```python
from build123d import *

# Parameters (mm, degrees)
F0_W        = 78
F0_H        = 38
F1_DEPTH    = 4
F2_W        = 78
F2_H        = 3
F3_DEPTH    = 81
F4_T1_DEPTH = 203
F5_R        = 31
F5_R_2      = 29.5
F6_DEPTH    = 27
F7_R        = 28.5
F8_DEPTH    = 3
F9_R        = 31
F10_DEPTH   = 2
F11_R       = 16
F12_DEPTH   = 2
F14_DEPTH   = 4


# Not quite as in the source:
# - a fillet or chamfer that OpenCascade refuses, or shapes differently, is made with other operations: its cross-section is extruded or revolved along the edge and cut away or added


with BuildPart() as f1:
    # F0 (on Top) → F1 (new body)
    with BuildSketch(Plane.XY):
        Rectangle(F0_W, F0_H)
    extrude(amount=F1_DEPTH)

    # F2 (on face) → F3 (join)
    with BuildSketch(Plane.XY.offset(4)):
        with Locations((0, 17.5)):
            Rectangle(F2_W, F2_H)
    extrude(amount=F3_DEPTH)

    # F4: fillet of radius 40 on 2 edges, made by hand

    # F4_s2 → F4_t1 (cut)
    with BuildSketch(Plane.XZ.offset(-119)):
        with BuildLine():
            ThreePointArc((39, 45), (27.2842712475, 73.2842712475), (-1, 85))
            Line((-1, 85), (39, 85))
            Line((39, 85), (39, 45))
        make_face()
        with BuildLine():
            ThreePointArc((-39, 45), (-27.2842712475, 73.2842712475), (1, 85))
            Line((1, 85), (-39, 85))
            Line((-39, 85), (-39, 45))
        make_face()
    extrude(amount=F4_T1_DEPTH, mode=Mode.SUBTRACT)

    # F5 (on face) → F6 (join)
    with BuildSketch(Plane(origin=(0, 19, 0), x_dir=(-1, 0, 0), z_dir=(0, 1, 0))):
        with Locations((0, 45.9753048304)):
            Circle(F5_R)
        with Locations((0, 45.9753048304)):
            Circle(F5_R_2, mode=Mode.SUBTRACT)
    extrude(amount=F6_DEPTH)

    # F7 (on face) → F8 (cut, through all)
    with BuildSketch(Plane(origin=(0, 19, 0), x_dir=(-1, 0, 0), z_dir=(0, 1, 0))):
        with Locations((0, 45.9753048304)):
            Circle(F7_R)
    extrude(amount=-F8_DEPTH, mode=Mode.SUBTRACT)

    # F9 (on face) → F10 (join)
    with BuildSketch(Plane(origin=(0, 46, 0), x_dir=(-1, 0, 0), z_dir=(0, 1, 0))):
        with Locations((0, 45.9753048304)):
            Circle(F9_R)
    extrude(amount=F10_DEPTH)

    # F11 (on face) → F12 (cut, through all)
    with BuildSketch(Plane(origin=(0, 48, 0), x_dir=(-1, 0, 0), z_dir=(0, 1, 0))):
        with Locations((0, 45.9753048304)):
            Circle(F11_R)
    extrude(amount=-F12_DEPTH, mode=Mode.SUBTRACT)

    # F13 (on face) → F14 (cut, through all)
    with BuildSketch(Plane.XY.offset(4)):
        with BuildLine():
            Line((29.2, -19), (33.7, -19))
            Line((33.7, -19), (33.7, -9))
            ThreePointArc((33.7, -9), (31.45, -11.25), (29.2, -9))
            Line((29.2, -9), (29.2, -19))
        make_face()
        with BuildLine():
            ThreePointArc((29.2, -9), (31.45, -11.25), (33.7, -9))
            Line((33.7, -9), (29.2, -9))
        make_face()
        with BuildLine():
            Line((29.2, -9), (33.7, -9))
            ThreePointArc((33.7, -9), (31.45, -6.75), (29.2, -9))
        make_face()
        with BuildLine():
            ThreePointArc((-29.2, -9), (-31.45, -6.75), (-33.7, -9))
            Line((-33.7, -9), (-29.2, -9))
        make_face()
        with BuildLine():
            ThreePointArc((-29.2, -9), (-31.45, -11.25), (-33.7, -9))
            Line((-33.7, -9), (-33.7, -19))
            Line((-33.7, -19), (-29.2, -19))
            Line((-29.2, -19), (-29.2, -9))
        make_face()
        with BuildLine():
            Line((-29.2, -9), (-33.7, -9))
            ThreePointArc((-33.7, -9), (-31.45, -11.25), (-29.2, -9))
        make_face()
    extrude(amount=-F14_DEPTH, mode=Mode.SUBTRACT)


solid = f1.part
```
The listing builds one solid part. Answer for the finished solid, in the listing's coordinates (mm). A direction names the side the tool comes from. Give positions to 0.01 mm unless a question says otherwise; leave off trailing zeros. Write each loop counter-clockwise with the first axis right and the second up, starting at its lowest first coordinate (ties: lowest second). Pieces come first, ordered by that corner, then holes. Notation, with made-up numbers: M -30.5,82.25 L -18.5,82.25 A35 cw -18.5,115.25 Z; hole C 16.5,31 d4. An arc over 180 degrees is marked long. Write each question's results on one line, items separated by ' | '.
Q1. A tool of negligible diameter and unlimited length cuts with its end or side. For faces 5 (the flat face through (-1, -1, 4)), 6 (the cylindrical face through (6.72, 33.297, 15.712)), 7 (the flat face through (33.7, -14, 2)), from which of +Z, -Z, +X, -X, +Y, -Y can it reach the whole face along a straight path? Write none if from no direction.
Output values:
face 5: +Z, +X, -X, -Y | face 6: +Y | face 7: +Z, -Z, -Y
Q2. Section B-B, the plane x = 3.5 is taken. Write down the section's boundary in (y, z).
Output values:
outline: M -19,0 L 19,0 L 19,15.17 L 48,15.17 L 48,30.36 L 46,30.36 L 46,16.68 L 19,16.68 L 19,17.69 L 16,17.69 L 16,4 L -19,4 Z; M 16,74.26 L 19,74.26 L 19,75.27 L 46,75.27 L 46,61.59 L 48,61.59 L 48,76.78 L 19,76.78 L 19,84.75 L 16,84.75 Z
Q3. For a pull along Y with two mould halves and no side action, classify faces 1 (the cylindrical face through (6.395, 32.311, 17.177)), 2 (the flat face through (-29.2, -14, 2)), 3 (the flat face through (-1, 16, 17)), 4 (the flat face through (-13, 48, 33)) as released by +Y, released by -Y, zero draft, split by the parting line, or undercut.
Output values:
face 1: undercut | face 2: zero draft | face 3: released by -Y | face 4: released by +Y
Q4. Consider L1, parallel to Z at x = 0, y = 46.7; L2, parallel to Z at x = 0, y = 17.05; L3, parallel to Z at x = 4, y = -15. Determine where each line is inside the solid, lowest interval first. Write a range as from..to.
Output values:
L1: 14.98..29.98, 61.98..76.98 | L2: 0..17.48, 74.48..84.99 | L3: 0..4
Q5. Section C-C, the plane y = -5.5 is taken. Write down the section's boundary in (x, z), then the cut area to 3 significant figures.
Output values:
outline: M -39,0 L 39,0 L 39,4 L -39,4 Z | area: 312 mm2
Q6. Flat-ended cylindrical pins translate along their axes: P1, Ø1.5, axis at x = 0.5, y = -11, coming from the +Z side; P2, Ø5, axis at x = 29, z = 21, coming from the +Y side; P3, Ø6, axis at x = -21, y = 27, coming from the +Z side. Find the tip coordinate at first contact, or state that the pin passes through.
Output values:
P1: z = 4 | P2: y = 19 | P3: z = 71.21
Q7. Section A-A, the plane z = 40.5 is taken. Write down the section's boundary in (x, y), then the cut area to 3 significant figures.
Output values:
outline: M -39,16 L -27.97,16 L -27.97,19 L -28.99,19 L -28.99,46 L -15.03,46 L -15.03,48 L -30.51,48 L -30.51,19 L -39,19 Z; M 15.03,46 L 28.99,46 L 28.99,19 L 27.97,19 L 27.97,16 L 39,16 L 39,19 L 30.51,19 L 30.51,48 L 15.03,48 Z | area: 210 mm2
Q8. Section D-D, the plane z = 24.5 is taken. Write down the section's boundary in (x, y), then the cut area to 3 significant figures.
Output values:
outline: M -39,16 L -18.74,16 L -18.74,19 L -20.23,19 L -20.23,46 L 20.23,46 L 20.23,19 L 18.74,19 L 18.74,16 L 39,16 L 39,19 L 22.36,19 L 22.36,48 L -22.36,48 L -22.36,19 L -39,19 Z | area: 326 mm2
